Autodesk Inventor part; units mm, degrees
ref_plane "YZ Plane" through (0, 0, 0) normal (1, 0, 0) x (0, 1, 0)
ref_plane "XZ Plane" through (0, 0, 0) normal (0, 1, 0) x (-1, 0, 0)
ref_plane "XY Plane" through (0, 0, 0) normal (0, 0, 1) x (1, 0, 0)
sketch "Esboço1" plane through (0, 0, 0) normal (0, 1, 0) x (-1, 0, 0)
  arc A0 (0, -805) -> (805, 0) centre (0, 0) ccw
  arc A1 (0, -845) -> (845, 0) centre (0, 0) ccw
  line L0 (805, 0) -> (845, 0)
  line L1 (0, -805) -> (0, -845)
  circle A2 centre (7.5, -815) radius 2.5
  circle A3 centre (7.5, -835) radius 2.5
  circle A4 centre (835, -7.5) radius 2.5
  circle A5 centre (815, -7.5) radius 2.5
  circle A6 centre (835, -7.5) radius 2.5
  circle A7 centre (815, -7.5) radius 2.5
  dimension "d0" = 805
  dimension "d1" = 845
  dimension "d2" = 5
  dimension "d3" = 5
  dimension "d4" = 20
  dimension "d6" = 7.5
  dimension "d7" = 5
  dimension "d8" = 5
  dimension "d9" = 7.5
  dimension "d10" = 10
  dimension "d11" = 20
  dimension "d13" = 7.5
  dimension "d14" = 7.5
  dimension "d15" = 10
extrude "Extrusão1" add sketch "Esboço1" along normal blind 3 contours A0 L0 A1 L1 | A2 | A3 | A4 | A5
sketch "Esboço4" plane through (0, 3, 0) normal (0, 1, 0) x (1, 0, 0)
  circle A0 centre (-825, 7.5) radius 2.5
  line L0 (-845, 0) -> (-805, 0)
  circle A1 centre (-7.5, 825) radius 2.5
  line L1 (0, 805) -> (0, 845)
  point P0 (0, 0)
  dimension "d19" = 5
  dimension "d22" = 7.5
  dimension "d25" = 5
  dimension "d26" = 7.5
  dimension "d44" = 20
  dimension "d45" = 20
hole "Furo1" at (-825, 3, -7.5) at (-7.5, 3, -825) direction (0, -1, 0) diameter 5 end through all
properties part number "Arco menor_CPY" material "Alumínio 6061"
CAD build for the part. Positions are in the model's coordinates, mm. Give positions to 0.01 mm unless a question says otherwise; leave off trailing zeros. Loops run counter-clockwise (first coordinate to the right, second up) from the corner with the lowest first, then second, coordinate; pieces in that order, holes last. Notation, with made-up numbers: M -32,-38.75 L -2,-38.75 A7 cw -2,-27.75 Z; hole C 66,-39.5 d10. An arc over 180 degrees is marked long. One line per question, with ' | ' between items. Start each with the question number.
1. Saw through at A-A on y = 2. Give the cut face in (x, z).
2. Saw through at B-B on z = -193. Give the cut face in (x, y).
3. Saw through at C-C on x = -284. Give the cut face in (y, z).
4. Flat gauge pin, fed straight in: pin 1 (1.5 mm diameter, centred on y = 1.5, z = -230, fed in from -X). Where does the tip first touch, or does it go through?
5. Probe L1, parallel to Z at x = -7.5, y = 1; L2, parallel to X at y = 1.75, z = -299.5. List the from-to ranges inside material, lowest first. Write a range as from..to.
Result sheet:
1) outline: M -845,0 A845 ccw 0,-845 L 0,-805 A805 cw -805,0 Z; hole C -825,-7.5 d5; hole C -7.5,-825 d5
2) outline: M -822.66,0 L -781.52,0 L -781.52,3 L -822.66,3 Z
3) outline: M 0,-795.84 L 3,-795.84 L 3,-753.24 L 0,-753.24 Z
4) pin 1: stops at x = -813.31
5) L1: z = -844.97..-827.5, -822.5..-804.97 | L2: x = -790.14..-747.21
